```python
from build123d import *

# Parameters (mm, degrees)
F1_DEPTH = 587.5
F2_R     = 25
F3_DEPTH = 7.5
F4_R     = 25
F5_DEPTH = 20
F6_W     = 16
F6_H     = 7.0096296601
F7_DEPTH = 13


with BuildPart() as f1:
    # F0 (on Front) → F1 (new body)
    with BuildSketch(Plane.XZ):
        with BuildLine():
            Line((98.404571414, 0), (119.5426846988, 10.4664480605))
            ThreePointArc((119.5426846988, 10.4664480605), (115.9110991547, 31.0582854123), (108.760225816, 50.7071324417))
            Line((108.760225816, 50.7071324417), (85.220858693, 49.202285707))
            Line((85.220858693, 49.202285707), (98.2937777555, 68.8355522572))
            ThreePointArc((98.2937777555, 68.8355522572), (84.8528137424, 84.8528137424), (68.8355522572, 98.2937777555))
            Line((68.8355522572, 98.2937777555), (49.202285707, 85.220858693))
            Line((49.202285707, 85.220858693), (50.7071324417, 108.760225816))
            ThreePointArc((50.7071324417, 108.760225816), (31.0582854123, 115.9110991547), (10.4664480605, 119.5426846988))
            Line((10.4664480605, 119.5426846988), (0, 98.404571414))
            Line((0, 98.404571414), (-10.4664480605, 119.5426846988))
            ThreePointArc((-10.4664480605, 119.5426846988), (-31.0582854123, 115.9110991547), (-50.7071324417, 108.760225816))
            Line((-50.7071324417, 108.760225816), (-49.202285707, 85.220858693))
            Line((-49.202285707, 85.220858693), (-68.8355522572, 98.2937777555))
            ThreePointArc((-68.8355522572, 98.2937777555), (-84.8528137424, 84.8528137424), (-98.2937777555, 68.8355522572))
            Line((-98.2937777555, 68.8355522572), (-85.220858693, 49.202285707))
            Line((-85.220858693, 49.202285707), (-108.760225816, 50.7071324417))
            ThreePointArc((-108.760225816, 50.7071324417), (-115.9110991547, 31.0582854123), (-119.5426846988, 10.4664480605))
            Line((-119.5426846988, 10.4664480605), (-98.404571414, 0))
            Line((-98.404571414, 0), (-119.5426846988, -10.4664480605))
            ThreePointArc((-119.5426846988, -10.4664480605), (-115.9110991547, -31.0582854123), (-108.760225816, -50.7071324417))
            Line((-108.760225816, -50.7071324417), (-85.220858693, -49.202285707))
            Line((-85.220858693, -49.202285707), (-98.2937777555, -68.8355522572))
            ThreePointArc((-98.2937777555, -68.8355522572), (-84.8528137424, -84.8528137424), (-68.8355522572, -98.2937777555))
            Line((-68.8355522572, -98.2937777555), (-49.202285707, -85.220858693))
            Line((-49.202285707, -85.220858693), (-50.7071324417, -108.760225816))
            ThreePointArc((-50.7071324417, -108.760225816), (-31.0582854123, -115.9110991547), (-10.4664480605, -119.5426846988))
            Line((-10.4664480605, -119.5426846988), (0, -98.404571414))
            Line((0, -98.404571414), (10.4664480605, -119.5426846988))
            ThreePointArc((10.4664480605, -119.5426846988), (31.0582854123, -115.9110991547), (50.7071324417, -108.760225816))
            Line((50.7071324417, -108.760225816), (49.202285707, -85.220858693))
            Line((49.202285707, -85.220858693), (68.8355522572, -98.2937777555))
            ThreePointArc((68.8355522572, -98.2937777555), (84.8528137424, -84.8528137424), (98.2937777555, -68.8355522572))
            Line((98.2937777555, -68.8355522572), (85.220858693, -49.202285707))
            Line((85.220858693, -49.202285707), (108.760225816, -50.7071324417))
            ThreePointArc((108.760225816, -50.7071324417), (115.9110991547, -31.0582854123), (119.5426846988, -10.4664480605))
            Line((119.5426846988, -10.4664480605), (98.404571414, 0))
        make_face()
    extrude(amount=F1_DEPTH)

    # F2 (on face) → F3 (join)
    with BuildSketch(Plane(origin=(0, 0, 0), x_dir=(-1, 0, 0), z_dir=(0, 1, 0))):
        Circle(F2_R)
    extrude(amount=F3_DEPTH)

    # F4 (on face) → F5 (join)
    with BuildSketch(Plane.XZ.offset(587.5)):
        Circle(F4_R)
    extrude(amount=F5_DEPTH)

    # F6 (on face) → F7 (cut)
    with BuildSketch(Plane.XZ.offset(607.5)):
        with Locations((0, 22.50481483)):
            Rectangle(F6_W, F6_H)
    extrude(amount=-F7_DEPTH, mode=Mode.SUBTRACT)


solid = f1.part
```
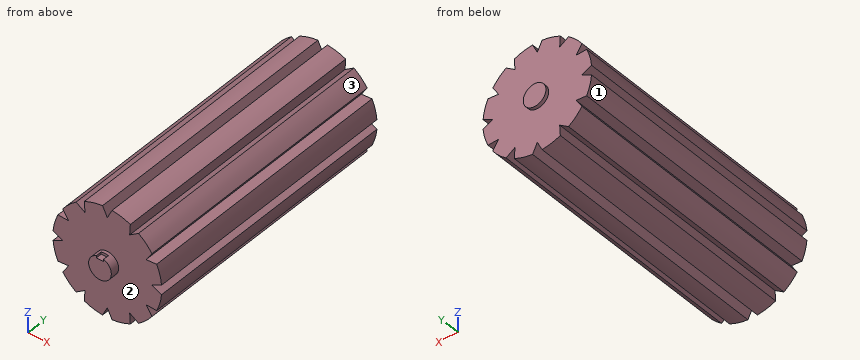
Check sheet for the modelled part. Datum: model origin and axes. Units: mm. Face numbers are marked on the shaded views. Round coordinates to 2 decimals unless told otherwise and drop trailing zeros.
1) Mould release check, pull along Z, two halves, no side actions. Record for the marked faces 1, 2 and 3: +Z half, -Z half, draft (parallel to the pull), parting line (faces both ways), or undercut.
2) Scan lines: line 1 (Y direction, x = 82, z = -61.5); line 2 (Z direction, x = -88, y = -384); line 3 (X direction, y = -302, z = -86). Record each from-to range of solid material in increasing order.
3) Go/stop test with flat-tipped pins: pin 1 Ø1.8 at (x, z) = (1.5, 23) entering from -Y; pin 2 Ø12 at (y, z) = (-501, -80.5) entering from -X; pin 3 Ø1.5 at (x, z) = (-52, -4.5) entering from +Y. Record where each tip stops, or that it passes through.
Result:
1. face 1: -Z half
1. face 2: draft
1. face 3: +Z half
2. line 1: y = -587.5 to 0
2. line 2: z = -81.58 to -53.38, -49.38 to 49.38, 53.38 to 81.58
2. line 3: x = -83.69 to -50.37, -49.25 to 49.25, 50.37 to 83.69
3. pin 1: stops at y = -594.5
3. pin 2: stops at x = -94.07
3. pin 3: stops at y = 0
